Source: CAD feature listing. Evaluate the final solid. Frame: model axes, mm. A direction names the side the tool comes from. Round coordinates to 2 decimals unless told otherwise and drop trailing zeros. Loops run counter-clockwise (first coordinate to the right, second up) from the corner with the lowest first, then second, coordinate; pieces in that order, holes last. Notation, with made-up numbers: (40, -3) - (53, -3) arc R32 ccw to (53, 31) - close; hole circle Ø2 at (-40, -27). An arc over 180 degrees is marked (long way). Write item = value, one per line. Start each with the question number.
from build123d import *

# Parameters (mm, degrees)
CUT_EXTRUDE1_REACH = 17.402
SKETCH2_W          = 3.052308152
SKETCH2_H          = 16.366405324


with BuildPart() as part:
    # Sketch1 → Revolve1 (revolve)
    with BuildSketch(Plane(origin=(0, 0, 0), x_dir=(0, 0, -1), z_dir=(1, 0, 0)), mode=Mode.PRIVATE) as revolve1_sk:
        Polygon((0, 4.125), (0, 5.25), (1, 5.25), (1, 6.5), (3.75, 10), (5.615100803, 10), (6.1, 7.25), (6.1, 5.175), (7, 5.175), (7, 4.125), align=None)
    revolve(revolve1_sk.sketch.rotate(Axis((0, 0, 0), (0, 0, -1)), 90), axis=Axis((0, 0, 0), (0, 0, -1)))

    # Cut-Extrude1: up to this cone (the profile starts inside it)
    cut_extrude1_end = Plane(origin=(0, 0, -6.1), z_dir=(0, 0, -1)).offset(-10.207141857) * Cone(1.273e-06, 52.309157025, 41.100050948, align=(Align.CENTER, Align.CENTER, Align.MIN), mode=Mode.PRIVATE)
    # Sketch2 → Cut-Extrude1 (cut, up to the surface)
    with BuildSketch(Plane(origin=(0, 0, -6.1), x_dir=(-1, 0, 0), z_dir=(0, 0, -1)), mode=Mode.PRIVATE) as cut_extrude1_sk1:
        with Locations((10.576154076, 0)):
            Rectangle(SKETCH2_W, SKETCH2_H)
    cut_extrude1_tool1 = extrude(cut_extrude1_sk1.sketch, amount=-CUT_EXTRUDE1_REACH, mode=Mode.PRIVATE) & cut_extrude1_end
    add(cut_extrude1_tool1.solids().sort_by_distance((-10.576154, 0, -6.1))[0], mode=Mode.SUBTRACT)
    # Sketch2 → Cut-Extrude1 (cut, up to the surface)
    with BuildSketch(Plane(origin=(0, 0, -6.1), x_dir=(-1, 0, 0), z_dir=(0, 0, -1)), mode=Mode.PRIVATE) as cut_extrude1_sk2:
        with Locations((-10.576154076, 0)):
            Rectangle(SKETCH2_W, SKETCH2_H)
    cut_extrude1_tool2 = extrude(cut_extrude1_sk2.sketch, amount=-CUT_EXTRUDE1_REACH, mode=Mode.PRIVATE) & cut_extrude1_end
    add(cut_extrude1_tool2.solids().sort_by_distance((10.576154, 0, -6.1))[0], mode=Mode.SUBTRACT)


solid = part.part
(1) Material intervals for line 1 along Y through (x, z) = (0, -4.25) (3 decimals); line 2 along Y through (x, z) = (3.25, -6.25); line 3 along X through (y, z) = (0.5, -3.25), sorted ascending. Write a range as from..to.
(2) Cut plane C-C (z = -4.25). Output: boundary loops of the cut face in (x, y) (3 decimals), and give its area (3 significant figures).
(3) Cut plane A-A (x = 0). Output: boundary loops of the cut face in (y, z) (3 decimals).
(4) Pin query (flat end, axial travel): P1, Ø3, axis at y = -1.5, z = -1.5, coming from the -X side. Return the tip coordinate at first contact, or that it passes through.
(5) Mould query, pull axis X, two halves, no side actions, for faces 1 (the face through (4, 2, 0)), 2 (the face through (-4.107, 3.149, -6.556)), 3 (the face through (-9.05, 0, -4)), 4 (the face through (4, -1, -3)). Classes: +X half, -X half, draft (parallel to the pull), parting line (faces both ways), or undercut.
(6) Cut plane D-D (z = -6.5). Output: boundary loops of the cut face in (x, y) (3 decimals).
(7) Cut plane B-B (y = 0). Output: boundary loops of the cut face in (x, z) (3 decimals), and give its area (3 significant figures).
(8) Access query for faces 5 (the face through (0, 10, -5)), 6 (the face through (-2, -5, -6.1)), 7 (the face through (5, -1.6, -0.5)). Directions: +Z, -Z, +X, -X, +Y, -Y. A direction counts if a zero-diameter tool reaches every point of the face in a straight line with its end or side. Return the directions, or none.
Solution:
q1.line_1 = -10..-4.125, 4.125..10
q1.line_2 = -4.03..-2.54, 2.54..4.03
q1.line_3 = -9.05..-4.09, 4.09..9.05
q2.outline = (-9.05, -4.254) arc R10 ccw to (9.05, -4.254) - (9.05, 4.254) arc R10 ccw to (-9.05, 4.254) - close; hole circle Ø8.25 at (0, 0)
q2.area = 250 mm^2
q3.outline = (-10, -5.615) - (-7.25, -6.1) - (-5.175, -6.1) - (-5.175, -7) - (-4.125, -7) - (-4.125, 0) - (-5.25, 0) - (-5.25, -1) - (-6.5, -1) - (-10, -3.75) - close; (4.125, -7) - (5.175, -7) - (5.175, -6.1) - (7.25, -6.1) - (10, -5.615) - (10, -3.75) - (6.5, -1) - (5.25, -1) - (5.25, 0) - (4.125, 0) - close
q4.P1 = -8.93
q5.face_1 = draft
q5.face_2 = parting line
q5.face_3 = -X half
q5.face_4 = undercut
q6.outline = circle Ø10.35 at (0, 0); hole circle Ø8.25 at (0, 0)
q7.outline = (-9.05, -5.783) - (-7.25, -6.1) - (-5.175, -6.1) - (-5.175, -7) - (-4.125, -7) - (-4.125, 0) - (-5.25, 0) - (-5.25, -1) - (-6.5, -1) - (-9.05, -3.004) - close; (4.125, -7) - (5.175, -7) - (5.175, -6.1) - (7.25, -6.1) - (9.05, -5.783) - (9.05, -3.004) - (6.5, -1) - (5.25, -1) - (5.25, 0) - (4.125, 0) - close
q7.area = 48.7 mm^2
q8.face_5 = +Z, -Z, +Y
q8.face_6 = -Z
q8.face_7 = +Z
